Design review of the part built by this model. Coordinates are the model's own, in mm. Face numbers are marked on the shaded views. A direction names the side the tool comes from. Round coordinates to 2 decimals unless told otherwise and drop trailing zeros. Loops run counter-clockwise (first coordinate to the right, second up) from the corner with the lowest first, then second, coordinate; pieces in that order, holes last. Notation, with made-up numbers: M 55.5,33 L 73.5,33 A18 cw 73.5,49 Z; hole C -30.75,21.25 d2. An arc over 180 degrees is marked long. Use a Markdown table: item, result.
from build123d import *

# Parameters (mm, degrees)
SKETCH1_R           = 3.3
BOSS_EXTRUDE1_DEPTH = 7
CUT_EXTRUDE1_DEPTH  = 66.038450166
SKETCH4_R           = 7
CUT_EXTRUDE2_DEPTH  = 2
FILLET1_R           = 2
FILLET2_R           = 1


with BuildPart() as part:
    # Sketch1 → Boss-Extrude1 (new body)
    with BuildSketch(Plane(origin=(0, 0, 0), x_dir=(1, 0, 0), z_dir=(0, 1, 0))):
        with BuildLine():
            Line((10.25, 18), (25, 26))
            Line((25, 26), (25, 41))
            Line((25, 41), (-25, 41))
            Line((-25, 41), (-25, 26))
            Line((-25, 26), (-10.25, 18))
            Line((-10.25, 18), (-10.25, 5))
            ThreePointArc((-10.25, 5), (-8.785533906, 1.464466094), (-5.25, 0))
            Line((-5.25, 0), (0, 0))
            Line((0, 0), (5.25, 0))
            ThreePointArc((5.25, 0), (8.785533906, 1.464466094), (10.25, 5))
            Line((10.25, 5), (10.25, 18))
        make_face()
        with Locations(Location((0, 9, 0), (0, 0, 270))):
            Circle(SKETCH1_R, mode=Mode.SUBTRACT)
    extrude(amount=BOSS_EXTRUDE1_DEPTH)

    # Sketch2 → Cut-Extrude1 (cut, through all)
    with BuildSketch(Plane(origin=(25, 0, 0), x_dir=(0, 0, -1), z_dir=(1, 0, 0))):
        Polygon((26, 7), (41, 0), (41, 7), align=None)
    extrude(amount=-CUT_EXTRUDE1_DEPTH, mode=Mode.SUBTRACT)

    # Sketch4 → Cut-Extrude2 (cut)
    with BuildSketch(Plane.XZ):
        with Locations(Location((0, -9, 0), (0, 0, 270))):
            Circle(SKETCH4_R)
    extrude(amount=-CUT_EXTRUDE2_DEPTH, mode=Mode.SUBTRACT)

    # Fillet1
    fillet1_edges = [part.edges().sort_by_distance(p)[0] for p in [
        (-10.25, 3.5, -18),
        (10.25, 3.5, -18),
    ]]
    fillet(fillet1_edges, radius=FILLET1_R)

    # Fillet2
    fillet2_edges = [part.edges().sort_by_distance(p)[0] for p in [
        (10.25, 7, -10.904757682),
        (-18.14823696, 7, -22.283789537),
        (-8.785533906, 7, -1.464466094),
        (0, 7, 0),
        (18.14823696, 7, -22.283789537),
        (-10.25, 7, -10.904757682),
        (10.531417421, 7, -17.832488442),
        (-10.531417421, 7, -17.832488442),
        (8.785533906, 7, -1.464466094),
    ]]
    fillet(fillet2_edges, radius=FILLET2_R)


solid = part.part
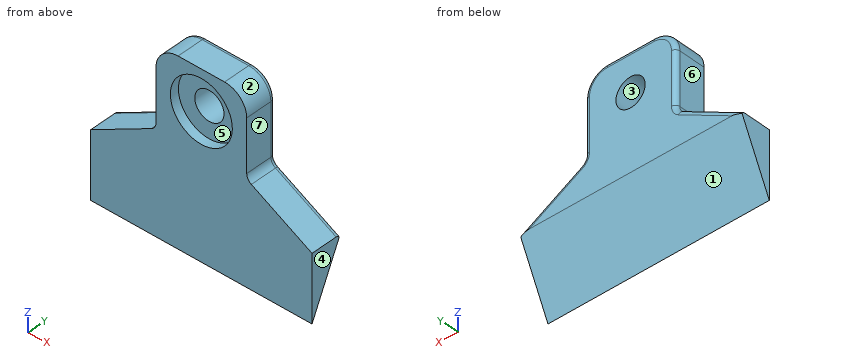
1. Wall thickness on line 1 along X through (y, z) = (1.4, -9); line 2 along X through (y, z) = (5.6, -9); line 3 along Z through (x, y) = (1, 1.75): over which ranges is each line inside the solid? List them lowest first. Write a range as from..to.
Check values:
| item | result |
|---|---|
| line 1 | x = -10.25..-7, 7..10.25 |
| line 2 | x = -10.25..-3.3, 3.3..10.25 |
| line 3 | z = -37.25..-15.93, -2.07..0 |
2. Take a section at D-D on z = -31. Give the boundary of the cut face in (x, y).
Check values:
| item | result |
|---|---|
| outline | M -25,0 L 25,0 L 25,4.67 L -25,4.67 Z |
3. The part is to be moulded in two halves that separate along X. For the marked faces 1, 2 and 3, say which applies: pulls with the +X half, pulls with the -X half, needs draft (parallel to the pull), parting line crosses it, or undercut.
Check values:
| item | result |
|---|---|
| face 1 | needs draft |
| face 2 | pulls with the +X half |
| face 3 | undercut |
4. Machinability: for the marked faces 4, 5, 6 and 7, which of the approach directions +Z, -Z, +X, -X, +Y, -Y give a long, thin tool a straight path to every point of the face, cutting with its end or side? Answer none if there is none.
Check values:
| item | result |
|---|---|
| face 4 | +Z, -Z, +X, +Y, -Y |
| face 5 | -Y |
| face 6 | +Z, -X, +Y, -Y |
| face 7 | +Z, +X, +Y, -Y |
5. Take a section at C-C on y = 3.5. Give the boundary of the cut face in (x, z).
Check values:
| item | result |
|---|---|
| outline | M -25,-33.5 L 25,-33.5 L 25,-26 L 11.3,-18.57 A2 cw 10.25,-16.81 L 10.25,-5 A5 ccw 5.25,0 L -5.25,0 A5 ccw -10.25,-5 L -10.25,-16.81 A2 cw -11.3,-18.57 L -25,-26 Z; hole C 0,-9 d6.6 |
6. Insertion check: pin 1 (2 mm diameter, centred on y = 4.5, z = -20, fed in from +X); pin 2 (4 mm diameter, centred on x = -1, z = -11, fed in from -Y); pin 3 (1.8 mm diameter, centred on y = 2, z = -11, fed in from -X). Each pin has a flat end and moves straight along its axis. Give the tip position at first contact, or say it passes through.
Check values:
| item | result |
|---|---|
| pin 1 | stops at x = 15.78 |
| pin 2 | stops at y = 2 |
| pin 3 | stops at x = -10.25 |
7. Take a section at B-B on x = 0. Give the boundary of the cut face in (y, z).
Check values:
| item | result |
|---|---|
| outline | M 0,-41 L 7,-26 L 7,-12.3 L 2,-12.3 L 2,-16 L 0,-16 Z; M 0,-2 L 2,-2 L 2,-5.7 L 7,-5.7 L 7,-1 A1 ccw 6,0 L 0,0 Z |
8. Take a section at A-A on z = -9. Give the boundary of the cut face in (x, y), and give its area (3 significant figures).
Check values:
| item | result |
|---|---|
| outline | M -10.25,0 L -7,0 L -7,2 L -3.3,2 L -3.3,7 L -9.25,7 A1 ccw -10.25,6 Z; M 3.3,2 L 7,2 L 7,0 L 10.25,0 L 10.25,6 A1 ccw 9.25,7 L 3.3,7 Z |
| area | 82.1 mm² |
